from build123d import *

# Parameters (mm, degrees)
EXTRUDE_1_DEPTH = 2


with BuildPart() as part:
    # 草图1 → 凸台-拉伸1 (new body)
    with BuildSketch(Plane(origin=(0, 0, 0), x_dir=(1, 0, 0), z_dir=(0, 1, 0))):
        Polygon((0, 5.75), (0, 0), (110, 0), (110, 30), (0, 30), (0, 15), align=None)
        with BuildLine():
            ThreePointArc((4, 2.75), (1, 5.75), (4, 8.75))
            Line((4, 8.75), (10, 8.75))
            ThreePointArc((10, 8.75), (13, 5.75), (10, 2.75))
            Line((10, 2.75), (4, 2.75))
        make_face(mode=Mode.SUBTRACT)
        with BuildLine():
            ThreePointArc((20, 2.75), (17, 5.75), (20, 8.75))
            Line((20, 8.75), (26, 8.75))
            ThreePointArc((26, 8.75), (29, 5.75), (26, 2.75))
            Line((26, 2.75), (20, 2.75))
        make_face(mode=Mode.SUBTRACT)
        with BuildLine():
            ThreePointArc((42, 1.5), (39, 4.5), (42, 7.5))
            Line((42, 7.5), (48, 7.5))
            ThreePointArc((48, 7.5), (51, 4.5), (48, 1.5))
            Line((48, 1.5), (42, 1.5))
        make_face(mode=Mode.SUBTRACT)
        with BuildLine():
            ThreePointArc((98, 1.5), (95, 4.5), (98, 7.5))
            Line((98, 7.5), (104, 7.5))
            ThreePointArc((104, 7.5), (107, 4.5), (104, 1.5))
            Line((104, 1.5), (98, 1.5))
        make_face(mode=Mode.SUBTRACT)
        with BuildLine():
            Line((10, 21.25), (4, 21.25))
            ThreePointArc((4, 21.25), (1, 24.25), (4, 27.25))
            Line((4, 27.25), (10, 27.25))
            ThreePointArc((10, 27.25), (13, 24.25), (10, 21.25))
        make_face(mode=Mode.SUBTRACT)
        with BuildLine():
            Line((26, 21.25), (20, 21.25))
            ThreePointArc((20, 21.25), (17, 24.25), (20, 27.25))
            Line((20, 27.25), (26, 27.25))
            ThreePointArc((26, 27.25), (29, 24.25), (26, 21.25))
        make_face(mode=Mode.SUBTRACT)
        with BuildLine():
            Line((48, 22.5), (42, 22.5))
            ThreePointArc((42, 22.5), (39, 25.5), (42, 28.5))
            Line((42, 28.5), (48, 28.5))
            ThreePointArc((48, 28.5), (51, 25.5), (48, 22.5))
        make_face(mode=Mode.SUBTRACT)
        with BuildLine():
            Line((104, 22.5), (98, 22.5))
            ThreePointArc((98, 22.5), (95, 25.5), (98, 28.5))
            Line((98, 28.5), (104, 28.5))
            ThreePointArc((104, 28.5), (107, 25.5), (104, 22.5))
        make_face(mode=Mode.SUBTRACT)
    extrude(amount=EXTRUDE_1_DEPTH)


solid = part.part
Here's how the part is built. I have some questions about the finished solid (model axes, mm). A direction names the side the tool comes from. Coordinates: 2 decimals unless noted, no trailing zeros. Write each loop counter-clockwise with the first axis right and the second up, starting at its lowest first coordinate (ties: lowest second). Pieces come first, ordered by that corner, then holes.
1) If we section it at A-A (x = 102): List the corners of the cut face in (y, z) for me.
Filled in:
outline: (0, -30) - (2, -30) - (2, -28.5) - (0, -28.5) - close; (0, -22.5) - (2, -22.5) - (2, -7.5) - (0, -7.5) - close; (0, -1.5) - (2, -1.5) - (2, 0) - (0, 0) - close
2) If we section it at B-B (z = -24.25): List the corners of the cut face in (x, y) for me, plus the area to 3 significant figures.
Filled in:
outline: (0, 0) - (1, 0) - (1, 2) - (0, 2) - close; (13, 0) - (17, 0) - (17, 2) - (13, 2) - close; (29, 0) - (39.27, 0) - (39.27, 2) - (29, 2) - close; (50.73, 0) - (95.27, 0) - (95.27, 2) - (50.73, 2) - close; (106.73, 0) - (110, 0) - (110, 2) - (106.73, 2) - close
area: 126 mm2
3) If I drill on line 1 (Z direction, x = 45.5, y = 1.95); line 2 (Z direction, x = 20.5, y = 0.7); line 3 (X direction, y = 1.85, z = -7.75), over which ranges is the centre line in solid material (lowest first)?
Filled in:
line 1: z = -30 to -28.5, -22.5 to -7.5, -1.5 to 0
line 2: z = -30 to -27.25, -21.25 to -8.75, -2.75 to 0
line 3: x = 0 to 1.76, 12.24 to 17.76, 28.24 to 110
4) Which directions (+Z, -Z, +X, -X, +Y, -Y) give clear straight access to the entire face, cutting with the end or side of a thin tool? Please do faces 1 (the face through (17, 1, -5.7)), 2 (the face through (54, 1, 0)).
Filled in:
face 1: +Y, -Y
face 2: +Z, +X, -X, +Y, -Y
5) I'm going to push a flat-ended pin straight in: pin 1 (0.6 mm diameter, centred on x = 24, y = 0.5, fed in from +Z). Where does the tip first touch, or does it pass through?
Filled in:
pin 1: stops at z = 0
6) Thinking about a two-plate mould opening in X: for faces 3 (the face through (54, 2, -15)), 4 (the face through (107, 1, -4.6)), which applies, +X half, -X half, draft (parallel to the pull), parting line (faces both ways), or undercut?
Filled in:
face 3: draft
face 4: undercut
7) If we section it at C-C (y = 0.95): Count the separate pieces of the cut face and the enclosed holes in it, plus the area to 3 significant figures.
Filled in:
separate pieces: 1
enclosed holes: 8
area: 2,790 mm2
